Source: CAD feature listing. Evaluate the final solid. Frame: model axes, mm. Round coordinates to 2 decimals unless told otherwise and drop trailing zeros. Write each loop counter-clockwise with the first axis right and the second up, starting at its lowest first coordinate (ties: lowest second). Pieces come first, ordered by that corner, then holes. Notation, with made-up numbers: M -38.5,44 L 17.5,44 A19 ccw 17.5,71 Z; hole C 63.25,66.5 d3. An arc over 180 degrees is marked long. Answer in a Markdown table with one row per item.
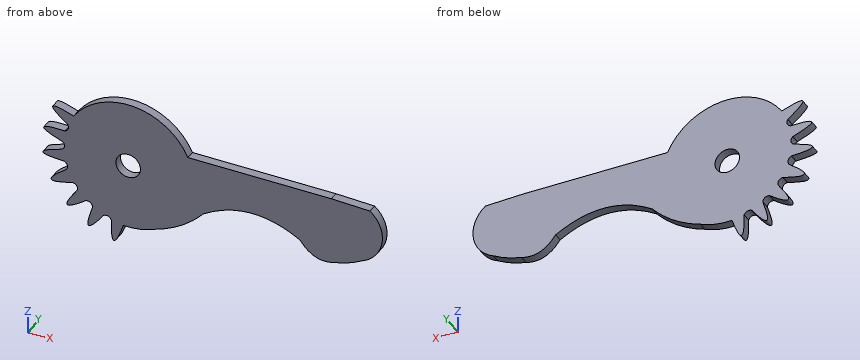
from build123d import *

# Parameters (mm, degrees)
SKETCH_1_R      = 3
EXTRUDE_1_DEPTH = 2.2


with BuildPart() as part:
    # 草图1 → 凸台-拉伸1 (new body)
    with BuildSketch(Plane(origin=(0, 0, 0), x_dir=(1, 0, 0), z_dir=(0, 1, 0))):
        with BuildLine():
            Line((14.611038219, -6.7), (49.690443214, -6.7))
            Line((49.690443214, -6.7), (59.14213471, -6.376451123))
            ThreePointArc((59.14213471, -6.376451123), (62.116009682, 1.036036266), (57.195522798, 7.327118086))
            add(Edge.make_bspline(
                [(50.347107534, 9.880159683), (52.761361064, 9.443859829), (55.044166152, 8.592845964), (57.195522798, 7.327118086)],
                knots=[0.288436631, 0.288436631, 0.288436631, 0.288436631, 1, 1, 1, 1], degree=3))
            add(Edge.make_bspline(
                [(41.984360593, 6.514151987), (43.667045792, 8.848960271), (46.317081673, 10.55679372), (49.303704664, 10.196073302), (50.347107534, 9.880159683)],
                knots=[0.090085046, 0.090085046, 0.090085046, 0.090085046, 0.520368733, 0.736118782, 0.736118782, 0.736118782, 0.736118782], degree=3))
            add(Edge.make_bspline(
                [(18.29395406, 7.037125327), (29.823970963, -0.449921726), (41.984360593, 6.514151987)],
                knots=[0, 0, 0, 1, 1, 1], degree=2))
            add(Edge.make_bspline(
                [(6.555128163, 14.676604942), (13.508953417, 12.492816522), (18.29395406, 7.037125327)],
                knots=[0, 0, 0, 1, 1, 1], degree=2))
            ThreePointArc((6.555128163, 14.676604942), (2.774471684, 15.832711225), (-1.174023286, 16.031035749))
            add(Edge.make_bspline(
                [(-4.132506817, 15.533667476), (-4.311159294, 25.643963381), (-1.174023286, 16.031035749)],
                knots=[0, 0, 0, 1, 1, 1], degree=2))
            add(Edge.make_bspline(
                [(-6.029547406, 14.900234761), (-4.764310754, 14.268430824), (-4.132506817, 15.533667476)],
                knots=[0, 0, 0, 1, 1, 1], degree=2))
            add(Edge.make_bspline(
                [(-8.69333509, 13.520294481), (-11.961242179, 23.089556901), (-6.029547406, 14.900234761)],
                knots=[0, 0, 0, 1, 1, 1], degree=2))
            add(Edge.make_bspline(
                [(-10.305043141, 12.336065974), (-8.907074862, 12.122326202), (-8.69333509, 13.520294481)],
                knots=[0, 0, 0, 1, 1, 1], degree=2))
            add(Edge.make_bspline(
                [(-12.417884822, 10.206300721), (-18.460681491, 18.31398895), (-10.305043141, 12.336065974)],
                knots=[0, 0, 0, 1, 1, 1], degree=2))
            add(Edge.make_bspline(
                [(-13.589217783, 8.585196439), (-12.192999161, 8.810082099), (-12.417884822, 10.206300721)],
                knots=[0, 0, 0, 1, 1, 1], degree=2))
            add(Edge.make_bspline(
                [(-15.07242577, 5.585196439), (-23.295073991, 11.517146599), (-13.589217783, 8.585196439)],
                knots=[0, 0, 0, 1, 1, 1], degree=2))
            add(Edge.make_bspline(
                [(-15.669039675, 3.585196439), (-14.412461062, 4.29933734), (-15.07242577, 5.585196439)],
                knots=[0, 0, 0, 1, 1, 1], degree=2))
            add(Edge.make_bspline(
                [(-16.063311706, 0.585196439), (-25.780917218, 3.388231532), (-15.669039675, 3.585196439)],
                knots=[0, 0, 0, 1, 1, 1], degree=2))
            add(Edge.make_bspline(
                [(-16.011582331, -1.414803561), (-15.037875075, -0.394118455), (-16.063311706, 0.585196439)],
                knots=[0, 0, 0, 1, 1, 1], degree=2))
            add(Edge.make_bspline(
                [(-15.455806267, -4.414803561), (-25.566384923, -4.736394924), (-16.011582331, -1.414803561)],
                knots=[0, 0, 0, 1, 1, 1], degree=2))
            add(Edge.make_bspline(
                [(-14.787919584, -6.299989859), (-14.179269776, -5.023453369), (-15.455806267, -4.414803561)],
                knots=[0, 0, 0, 1, 1, 1], degree=2))
            add(Edge.make_bspline(
                [(-13.318124412, -9), (-22.835991784, -12.431149783), (-14.787919584, -6.299989859)],
                knots=[0, 0, 0, 1, 1, 1], degree=2))
            ThreePointArc((-13.318124412, -9), (1.319244681, -16.019738803), (14.611038219, -6.7))
        make_face()
        with Locations(Location((0, 0, 0), (0, 0, 270))):
            Circle(SKETCH_1_R, mode=Mode.SUBTRACT)
    extrude(amount=EXTRUDE_1_DEPTH)


solid = part.part
Q1. Material intervals for probe 1 along Z at (x, y) = (-16, 0.5); probe 2 along X at (y, z) = (0.55, 0); probe 3 along Z at (x, y) = (20, 0.3), sorted ascending.
Solutions:
| item | result |
|---|---|
| probe 1 | z = -9.24 to -6.27, -3.58 to -0.52, 1.4 to 4.43, 7.25 to 9.88 |
| probe 2 | x = -15.63 to -3, 3 to 62.2 |
| probe 3 | z = -6.01 to 6.7 |
Q2. Section A-A (x = 0). Return loops of the section in (y, z).
Solutions:
| item | result |
|---|---|
| outline | M 0,-16.07 L 2.2,-16.07 L 2.2,-3 L 0,-3 Z; M 0,3 L 2.2,3 L 2.2,16.07 L 0,16.07 Z |
Q3. Contact query for a flat-ended pin moving along its axis: pin 1 Ø5.5 at (x, z) = (0, 0) entering from +Y (1 decimal). Output: stop coordinate, or through.
Solutions:
| item | result |
|---|---|
| pin 1 | passes through |
Q4. Section B-B (z = 11.5). Return loops of the section in (x, y).
Solutions:
| item | result |
|---|---|
| outline | M -11.23,0 L 11.23,0 L 11.23,2.2 L -11.23,2.2 Z |
